```python
from build123d import *

# Parameters (mm, degrees)
SKETCH1_R           = 8
SKETCH1_R_2         = 4
BOSS_EXTRUDE2_DEPTH = 10
SKETCH1_4_R         = 8
CUT_EXTRUDE1_DEPTH  = 4
SKETCH1_6_R         = 4
CUT_EXTRUDE2_DEPTH  = 24
SKETCH2_R           = 4
BOSS_EXTRUDE3_DEPTH = 10
SKETCH3_R           = 4
BOSS_EXTRUDE4_DEPTH = 10
CHAMFER1_SIZE       = 1


with BuildPart() as part:
    # Sketch1 → Boss-Extrude2 (new body)
    with BuildSketch(Plane.XY):
        with BuildLine():
            ThreePointArc((-28, 81.967733539), (0, 88), (28, 81.967733539))
            Line((28, 81.967733539), (28, 0))
            Line((28, 0), (-28, 0))
            Line((-28, 0), (-28, 81.967733539))
        make_face()
        with Locations((0, 20)):
            Circle(SKETCH1_R, mode=Mode.SUBTRACT)
        with BuildLine():
            ThreePointArc((-15.529142706, 77.955549577), (-18.357569831, 73.056570092), (-13.458590345, 70.228142967))
            ThreePointArc((-13.458590345, 70.228142967), (0, 72), (13.458590345, 70.228142967))
            ThreePointArc((13.458590345, 70.228142967), (18.357569831, 73.056570092), (15.529142706, 77.955549577))
            ThreePointArc((15.529142706, 77.955549577), (0, 80), (-15.529142706, 77.955549577))
        make_face(mode=Mode.SUBTRACT)
        with Locations((0, 20)):
            Circle(SKETCH1_R)
        with Locations((0, 20)):
            Circle(SKETCH1_R_2, mode=Mode.SUBTRACT)
        with Locations((0, 20)):
            Circle(SKETCH1_R_2)
    extrude(amount=-BOSS_EXTRUDE2_DEPTH)

    # Sketch1_4 → Cut-Extrude1 (cut)
    with BuildSketch(Plane.XY):
        with Locations((0, 20)):
            Circle(SKETCH1_4_R)
    extrude(amount=-CUT_EXTRUDE1_DEPTH, mode=Mode.SUBTRACT)

    # Sketch1_6 → Cut-Extrude2 (cut)
    with BuildSketch(Plane.XY):
        with Locations((0, 20)):
            Circle(SKETCH1_6_R)
    extrude(amount=-CUT_EXTRUDE2_DEPTH, mode=Mode.SUBTRACT)

    # Sketch2 → Boss-Extrude3 (add)
    with BuildSketch(Plane.ZY.offset(28)):
        Polygon((0, 64), (0, 0), (20, 0), (20, 54), align=None)
        with Locations(Location((10, 44, 0), (0, 0, 270))):
            Circle(SKETCH2_R, mode=Mode.SUBTRACT)
    extrude(amount=-BOSS_EXTRUDE3_DEPTH)

    # Sketch3 → Boss-Extrude4 (add)
    with BuildSketch(Plane(origin=(28, 0, 0), x_dir=(0, 0, -1), z_dir=(1, 0, 0))):
        Polygon((-20, 54), (-20, 0), (0, 0), (0, 64), align=None)
        with Locations(Location((-10, 44, 0), (0, 0, 270))):
            Circle(SKETCH3_R, mode=Mode.SUBTRACT)
    extrude(amount=-BOSS_EXTRUDE4_DEPTH)

    # Chamfer1
    chamfer1_edges = [part.edges().sort_by_distance(p)[0] for p in [
        (28, 72.98386677, 0),
        (0, 88, 0),
        (-28, 72.98386677, 0),
        (-28, 27, 20),
        (-28, 59, 10),
        (28, 27, 20),
        (28, 59, 10),
    ]]
    chamfer(chamfer1_edges, length=CHAMFER1_SIZE)


solid = part.part
```
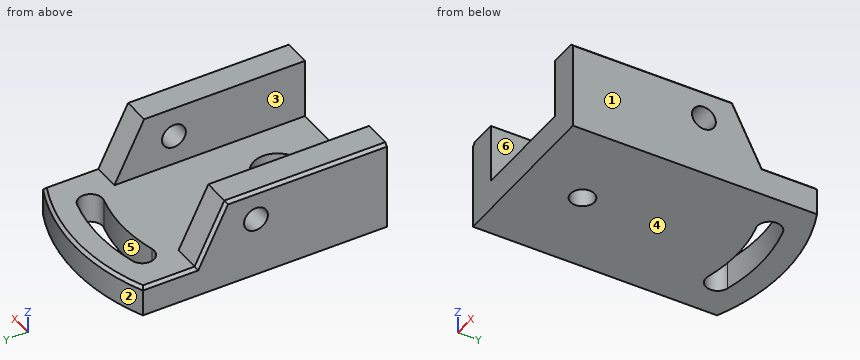
For this review, take the finished solid that the model builds, in its own axes (mm). Face numbers are marked on the shaded views. A direction names the side the tool comes from. Coordinates: 2 decimals unless noted, no trailing zeros. Write each loop counter-clockwise with the first axis right and the second up, starting at its lowest first coordinate (ties: lowest second). Pieces come first, ordered by that corner, then holes. Notation, with made-up numbers: (29.5, -18.75) - (52.5, -18.75) arc R6 ccw to (52.5, -8.75) - close; hole circle Ø7 at (69.25, 57.5). An arc over 180 degrees is marked (long way). Answer in a Markdown table with one row per item. Add a question column.
Q1. We need section A-A, the plane y = 44. State the section outline as (x, z) points.
Q2. We need section D-D, the plane z = 4.5. State the section outline as (x, y) points, and give its area (3 significant figures).
Q3. We need section B-B, the plane x = 0. State the section outline as (y, z) points.
Q4. Tool access review of the marked faces 4, 5 and 6: name each direction out of +Z, -Z, +X, -X, +Y, -Y from which nothing blocks a thin tool from reaching the whole face with its end or side.
Q5. For P1, Ø13, axis at x = 0, y = 20, coming from the +Z side; P2, Ø8, axis at x = -2.5, y = 61, coming from the +Z side; P3, Ø6.5, axis at x = 0, y = 20, coming from the -Z side; P4, Ø8, axis at x = 7.5, z = -0.5, coming from the +Y side, all flat-tipped, find the tip position at first contact; note any pin that passes through.
Q6. For probe 1 along Y at (x, z) = (0, -6.3); probe 2 along Y at (x, z) = (0, -2.3); probe 3 along X at (y, z) = (24, 18), list the stretches that pass through material, from the lowest coordinate up.
Q7. Draft analysis for pull direction X (two halves, no side actions). For the marked faces 1, 2 and 3, state which applies: +X half, -X half, draft (parallel to the pull), parting line (faces both ways), or undercut.
Q8. We need section C-C, the plane y = 20. State the section outline as (x, z) points, and give its area (3 significant figures).
Answer list:
| question | item | result |
|---|---|---|
| 1 | outline | (-28, -10) - (28, -10) - (28, 6) - (18, 6) - (18, 0) - (-18, 0) - (-18, 6) - (-28, 6) - close; (-28, 14) - (-18, 14) - (-18, 20) - (-27, 20) - (-28, 19) - close; (18, 14) - (28, 14) - (28, 19) - (27, 20) - (18, 20) - close |
| 2 | outline | (-28, 0) - (-18, 0) - (-18, 61.75) - (-27, 61.75) - (-28, 60.63) - close; (18, 0) - (28, 0) - (28, 60.63) - (27, 61.75) - (18, 61.75) - close |
| 2 | area | 1,230 mm2 |
| 3 | outline | (0, -10) - (16, -10) - (16, -4) - (12, -4) - (12, 0) - (0, 0) - close; (24, -10) - (72, -10) - (72, 0) - (28, 0) - (28, -4) - (24, -4) - close; (80, -10) - (88, -10) - (88, -1) - (87, 0) - (80, 0) - close |
| 4 | face 4 | -Z, +X, -X, +Y, -Y |
| 4 | face 5 | +Z, -Z |
| 4 | face 6 | +Z, +Y, -Y |
| 5 | P1 | stops at z = -4 |
| 5 | P2 | stops at z = 0 |
| 5 | P3 | passes through |
| 5 | P4 | stops at y = 87.91 |
| 6 | probe 1 | y = 0 to 16, 24 to 72, 80 to 88 |
| 6 | probe 2 | y = 0 to 12, 28 to 72, 80 to 88 |
| 6 | probe 3 | x = -28 to -18, 18 to 28 |
| 7 | face 1 | +X half |
| 7 | face 2 | parting line |
| 7 | face 3 | undercut |
| 8 | outline | (-28, -10) - (-4, -10) - (-4, -4) - (-8, -4) - (-8, 0) - (-18, 0) - (-18, 20) - (-27, 20) - (-28, 19) - close; (4, -10) - (28, -10) - (28, 19) - (27, 20) - (18, 20) - (18, 0) - (8, 0) - (8, -4) - (4, -4) - close |
| 8 | area | 847 mm2 |
